```python
from build123d import *

# Parameters (mm, degrees)
SKETCH1_W             = 19.05
SKETCH1_H             = 19.05
SKETCH1_W_2           = 15.875
SKETCH1_H_2           = 15.875
TUBE_DEPTH            = 758.9266
SKETCH2_R             = 2.8956
SIDE_WALL_HOLES_DEPTH = 20.05
LPATTERN1_COUNT       = 4
LPATTERN1_PITCH       = 210.574466667
SKETCH3_R             = 2.8956
REARWALLHOLES_DEPTH   = 20.05
LPATTERN2_COUNT       = 4
LPATTERN2_PITCH       = 227.084466667


with BuildPart() as part:
    # Sketch1 → Tube (new body)
    with BuildSketch(Plane(origin=(0, 0, 0), x_dir=(1, 0, 0), z_dir=(0, 1, 0))):
        Rectangle(SKETCH1_W, SKETCH1_H)
        Rectangle(SKETCH1_W_2, SKETCH1_H_2, mode=Mode.SUBTRACT)
    extrude(amount=TUBE_DEPTH)

    # Sketch2 → Side Wall Holes (cut, through all)
    with BuildSketch(Plane.XY.offset(9.525)):
        with Locations((0, 695.325)):
            Circle(SKETCH2_R)
    side_wall_holes = extrude(amount=-SIDE_WALL_HOLES_DEPTH, mode=Mode.SUBTRACT)

    # LPattern1: Side Wall Holes ×4
    with Locations(*[(0, -i * LPATTERN1_PITCH, 0) for i in range(1, LPATTERN1_COUNT)]):
        add(side_wall_holes, mode=Mode.SUBTRACT)

    # Sketch3 → RearWallHoles (cut, through all)
    with BuildSketch(Plane.ZY.offset(9.525)):
        with Locations((0, 720.09)):
            Circle(SKETCH3_R)
    rearwallholes = extrude(amount=-REARWALLHOLES_DEPTH, mode=Mode.SUBTRACT)

    # LPattern2: RearWallHoles ×4
    with Locations(*[(0, -i * LPATTERN2_PITCH, 0) for i in range(1, LPATTERN2_COUNT)]):
        add(rearwallholes, mode=Mode.SUBTRACT)


solid = part.part
```
Geometry: final body of the model. Coordinates: model frame, mm. A direction names the side the tool comes from. Give positions to 0.01 mm unless a question says otherwise; leave off trailing zeros. Order: outer loops, then holes, each group sorted by start corner. A loop starts at its lowest first (then second) coordinate and runs counter-clockwise, first axis right, second up. Notation, with made-up numbers: (77, 6.5) -> (99, 6.5) arc R11 ccw to (99, 20.5) -> close; hole circle Ø2 at (-5, 47). An arc over 180 degrees is marked (long way). Write each question's results on one line, items separated by ' | '. Start each with the question number.
1) Set-up query: faces 5 (the flat face through (0, 374, 7.938)), 6 (the flat face through (-9, 0, 0)). Return all of +Z, -Z, +X, -X, +Y, -Y with unobstructed straight access to the full face (end or side cutting, diameter ignored); none if empty.
2) Section B-B (z = 0). Count the separate pieces of the cut face and the enclosed holes in it, then the cut area to 3 significant figures.
3) Draft query along Z for faces 1 (the flat face through (9.525, 374, 0)), 2 (the flat face through (0, 374, 9.525)), 3 (the flat face through (-7.938, 374, 0)), 4 (the flat face through (0, 374, -7.938)). Return one class per face: pulls with the +Z half, pulls with the -Z half, needs draft (parallel to the pull), parting line crosses it, or undercut.
4) Section A-A (y = 180.5). Return loops of the section in (x, z) (1 decimal).
5) First-contact query: pin 1 (9.5 mm diameter, centred on x = 0, y = 274.18, fed in from -Z) (3 decimals). Flat tip, straight axial feed; report the tip coordinate or a pass-through.
6) Line query: line 1 (Y direction, x = -9.1, z = 0); line 2 (Y direction, x = 0, z = -8.4); line 3 (X direction, y = 394, z = 6.5) (1 decimal). Output: solid intervals per line, ascending. Write a range as from..to.
Calculated:
1) face 5: +Y, -Y | face 6: +Z, -Z, +X, -X, -Y
2) separate pieces: 10 | enclosed holes: 0 | area: 2,340 mm2
3) face 1: needs draft | face 2: pulls with the +Z half | face 3: undercut | face 4: undercut
4) outline: (-9.5, -9.5) -> (9.5, -9.5) -> (9.5, 9.5) -> (-9.5, 9.5) -> close; hole (-7.9, -7.9) -> (7.9, -7.9) -> (7.9, 7.9) -> (-7.9, 7.9) -> close
5) pin 1: z = -9.525
6) line 1: 0..35.94, 41.73..263.03, 268.82..490.11, 495.9..717.19, 722.99..758.93 | line 2: 0..60.71, 66.5..271.28, 277.07..481.85, 487.65..692.43, 698.22..758.93 | line 3: -9.5..-7.9, 7.9..9.5
